```python
from build123d import *

# Parameters (mm, degrees)
SKETCH_1_W      = 50
SKETCH_1_H      = 47
EXTRUDE_1_DEPTH = 2
EXTRUDE_2_DEPTH = 8
SKETCH_3_W      = 24
SKETCH_3_H      = 3
EXTRUDE_3_DEPTH = 10


with BuildPart() as part:
    # Эскиз1 → Бобышка-Вытянуть1 (new body)
    with BuildSketch(Plane(origin=(0, 0, 0), x_dir=(1, 0, 0), z_dir=(0, 1, 0))):
        with Locations((25, 23.5)):
            Rectangle(SKETCH_1_W, SKETCH_1_H)
    extrude(amount=EXTRUDE_1_DEPTH)

    # Эскиз2 → Бобышка-Вытянуть2 (add)
    with BuildSketch(Plane(origin=(0, 2, 0), x_dir=(1, 0, 0), z_dir=(0, 1, 0))):
        Polygon((25, 37), (13, 37), (13, 33), (37, 33), (37, 37), align=None)
    extrude(amount=EXTRUDE_2_DEPTH)

    # Эскиз3 → Бобышка-Вытянуть3 (add)
    with BuildSketch(Plane.XY.offset(-33)):
        with Locations((25, 8.5)):
            Rectangle(SKETCH_3_W, SKETCH_3_H)
    extrude(amount=EXTRUDE_3_DEPTH)


solid = part.part
```
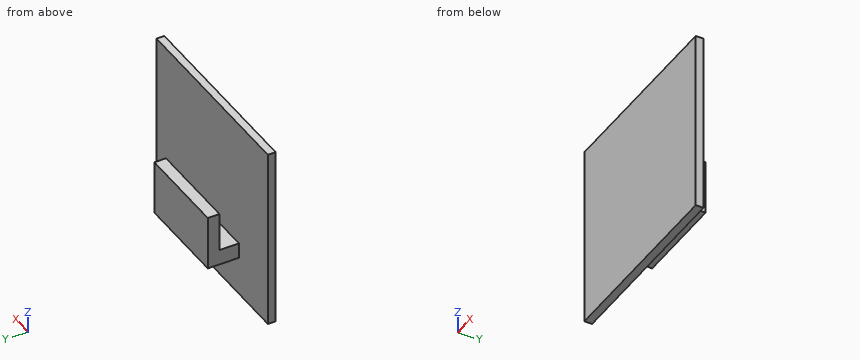
Geometry check sheet. Reference: the model listing, model coordinates, mm. Coordinates: 2 decimals unless noted, no trailing zeros. Order: outer loops, then holes, each group sorted by start corner. A loop starts at its lowest first (then second) coordinate and runs counter-clockwise, first axis right, second up.
Q1. Sectioned sample at C-C on y = 8.25. Record the cut outline in (x, z), and give its area (3 significant figures).
Reply:
outline: (13, -37) - (37, -37) - (37, -23) - (13, -23) - close
area: 336 mm2
Q2. Sectioned sample at A-A on x = 35.5. Record the cut outline in (y, z).
Reply:
outline: (0, -47) - (2, -47) - (2, -37) - (10, -37) - (10, -23) - (7, -23) - (7, -33) - (2, -33) - (2, 0) - (0, 0) - close
Q3. Sectioned sample at B-B on z = -21. Record the cut outline in (x, y), and give its area (3 significant figures).
Reply:
outline: (0, 0) - (50, 0) - (50, 2) - (0, 2) - close
area: 100 mm2
Q4. Depth check by flat-ended pin: pin 1 Ø2.5 at (x, y) = (22.5, 3.5) entering from +Z; pin 2 Ø3 at (x, z) = (43, -11.5) entering from -Y; pin 3 Ø3.5 at (x, y) = (22.5, 8.5) entering from +Z; pin 4 Ø6 at (x, z) = (41.5, -19) entering from +Y. Enter the tip coordinate at first touch or a pass-through.
Reply:
pin 1: stops at z = -33
pin 2: stops at y = 0
pin 3: stops at z = -23
pin 4: stops at y = 2
Q5. Thickness scan on probe 1 along Y at (x, z) = (29, -19.5); probe 2 along Z at (x, y) = (30, 3); probe 3 along Z at (x, y) = (17, 7.5). Record the ranges inside material, lowest first.
Reply:
probe 1: y = 0 to 2
probe 2: z = -37 to -33
probe 3: z = -37 to -23
